Part model, mm, in its own coordinate system. A direction names the side the tool comes from. Give positions to 0.01 mm unless a question says otherwise; leave off trailing zeros. Order: outer loops, then holes, each group sorted by start corner. A loop starts at its lowest first (then second) coordinate and runs counter-clockwise, first axis right, second up.
1. Slice it at D-D on y = -2.75. List the corners of the cut face in (x, z).
2. Slice it at C-C on z = 24.5. List the corners of the cut face in (x, y).
3. Mould opens along X. For faces 3 (the cylindrical face through (-0.661, 5.037, 3.757)), 4 (the flat face through (-3.81, -9, 35)), 5 (the flat face through (-5.2, 0.6, 7.62)) say: +X half, -X half, draft (parallel to the pull), parting line (faces both ways), or undercut.
4. Which spindle directions (+Z, -Z, +X, -X, +Y, -Y) get a long thin tool onto all of the face, cutting with end or side? Do faces 1 (the cylindrical face through (0.279, 7.615, 3.757)), 2 (the flat face through (0, -6.599, 39)). Say none if no direction does.
5. Slice it at B-B on z = 6.5. List the corners of the cut face in (x, y), and give its area (3 significant figures).
6. Probe line 1 (X direction, y = -10.16, z = 5.25); line 2 (Y direction, x = 0, z = 35.5); line 3 (Z direction, x = -6.5, y = 0.75). List the from-to ranges inside material, lowest first.
7. Slice it at A-A on y = 0. List the corners of the cut face in (x, z).
8. Drop flat-ended pins along their axis: pin 1 Ø4 at (y, z) = (-9.5, 46) entering from +X; pin 2 Ø5.5 at (y, z) = (-9, 39.5) entering from -X; pin 3 Ø3 at (x, y) = (2.5, -4.5) entering from +Z; pin 4 Ø4 at (x, y) = (0, -10.16) entering from -Z. Give the stop position or say it passes through.
from build123d import *

# Parameters (mm, degrees)
F0_R     = 7.62
F0_R_2   = 5.08
F1_DEPTH = 7.62
F3_DEPTH = 7.62
F4_R     = 2.54
F5_R     = 2.54
F6_DEPTH = 63.5


with BuildPart() as f1:
    # F0 (on Top) → F1 (new body)
    with BuildSketch(Plane.XY):
        Circle(F0_R)
        Circle(F0_R_2, mode=Mode.SUBTRACT)
    extrude(amount=F1_DEPTH)

    # F2 (on face) → F3 (join)
    with BuildSketch(Plane.XY.offset(7.62)):
        with BuildLine():
            ThreePointArc((3.7e-09, -7.62), (-1.9722011219, -7.3603547968), (-3.81, -6.5991135768))
            Line((-3.81, -6.5991135768), (-3.81, -13.97))
            Line((-3.81, -13.97), (3.81, -13.97))
            Line((3.81, -13.97), (3.81, -6.5991135768))
            ThreePointArc((3.81, -6.5991135768), (1.9722011255, -7.3603547958), (3.7e-09, -7.62))
        make_face()
        with BuildLine():
            ThreePointArc((2.54, -10.16), (-1.7960512255, -11.9560512229), (3.7e-09, -7.62))
            ThreePointArc((3.7e-09, -7.62), (1.7960512255, -8.3639487771), (2.54, -10.16))
        make_face(mode=Mode.SUBTRACT)
        with BuildLine():
            Line((0, -5.08), (-3.81, -5.08))
            Line((-3.81, -5.08), (-3.81, -6.5991135768))
            ThreePointArc((-3.81, -6.5991135768), (-1.9722011219, -7.3603547968), (3.7e-09, -7.62))
            ThreePointArc((3.7e-09, -7.62), (1.9722011255, -7.3603547958), (3.81, -6.5991135768))
            Line((3.81, -6.5991135768), (3.81, -5.08))
            Line((3.81, -5.08), (0, -5.08))
        make_face()
    extrude(amount=-F3_DEPTH)

    # F4
    f4_edges = [f1.edges().sort_by_distance(p)[0] for p in [
        (3.81, -13.97, 3.81),
        (-3.81, -13.97, 3.81),
    ]]
    fillet(f4_edges, radius=F4_R)

    # F5 (on face) → F6 (join)
    with BuildSketch(Plane.XY.offset(7.62)):
        with BuildLine():
            Line((3.81, -6.5991135768), (-3.81, -6.5991135768))
            Line((-3.81, -6.5991135768), (-3.81, -11.43))
            ThreePointArc((-3.81, -11.43), (-3.0660512242, -13.2260512242), (-1.27, -13.97))
            Line((-1.27, -13.97), (1.27, -13.97))
            ThreePointArc((1.27, -13.97), (3.0660512242, -13.2260512242), (3.81, -11.43))
            Line((3.81, -11.43), (3.81, -6.5991135768))
        make_face()
        with Locations((0, -10.16)):
            Circle(F5_R, mode=Mode.SUBTRACT)
    extrude(amount=F6_DEPTH)


solid = f1.part
Data:
1. outline: (-7.11, 0) - (-4.27, 0) - (-4.27, 7.62) - (-7.11, 7.62) - close; (4.27, 0) - (7.11, 0) - (7.11, 7.62) - (4.27, 7.62) - close
2. outline: (-3.81, -11.43) arc R2.54 ccw to (-1.27, -13.97) - (1.27, -13.97) arc R2.54 ccw to (3.81, -11.43) - (3.81, -6.6) - (-3.81, -6.6) - close; hole circle Ø5.08 at (0, -10.16)
3. face 3: undercut
3. face 4: -X half
3. face 5: draft
4. face 1: +Z, -Z
4. face 2: +Z, +X, -X, +Y
5. outline: (-3.81, -11.43) arc R2.54 ccw to (-1.27, -13.97) - (1.27, -13.97) arc R2.54 ccw to (3.81, -11.43) - (3.81, -6.6) arc R7.62 ccw (long way) to (-3.81, -6.6) - close; hole circle Ø10.16 at (0, 0); hole circle Ø5.08 at (0, -10.16)
5. area: 129 mm2
6. line 1: x = -3.81 to -2.54, 2.54 to 3.81
6. line 2: y = -13.97 to -12.7, -7.62 to -6.6
6. line 3: z = 0 to 7.62
7. outline: (-7.62, 0) - (-5.08, 0) - (-5.08, 7.62) - (-7.62, 7.62) - close; (5.08, 0) - (7.62, 0) - (7.62, 7.62) - (5.08, 7.62) - close
8. pin 1: stops at x = 3.81
8. pin 2: stops at x = -3.81
8. pin 3: stops at z = 7.62
8. pin 4: passes through
